Build history of the part. All positions in model axes, mm. A direction names the side the tool comes from. Coordinates: 2 decimals unless noted, no trailing zeros. Write each loop counter-clockwise with the first axis right and the second up, starting at its lowest first coordinate (ties: lowest second). Pieces come first, ordered by that corner, then holes. Notation, with made-up numbers: (-31.75, 19) -> (0.25, 19) arc R20 ccw to (0.25, 39) -> close; hole circle Ø7 at (-36, -9). An arc over 180 degrees is marked (long way). Write each question's results on one line, items separated by ' | '. Start each with the question number.
Q1. Saw through at B-B on z = 31. Give the cut face in (x, y), and give its area (3 significant figures).
Q2. Drop a flat-ended pin along its axis: pin 1 Ø8 at (x, z) = (22, -3) entering from -Y. Give the stop position or say it passes through.
Q3. Two-plate mould, pull along Z, no slides. Class faces 1 (the face through (-18.07, 1.48, -27.26)), 2 (the face through (-43, 26, -43)), 3 (the face through (-41, 29, 41)): released by +Z, released by -Z, zero draft, split by the parting line, or undercut.
Q4. Tool access for faces 4 (the face through (39.3, 27.5, -40.8)), 5 (the face through (-18.583, 1.479, 27.776)), 6 (the face through (-27.776, 1.479, -18.583)): list every direction of +Z, -Z, +X, -X, +Y, -Y with a clear straight run to the whole face (end or side of a thin tool).
Q5. Saw through at C-C on x = 41.25. Give the cut face in (y, z), and give its area (3 significant figures).
Q6. Drill centre lines: line 1 (Z direction, x = -41, y = 3.75); line 2 (Y direction, x = -14, z = 5); line 3 (X direction, y = 19.75, z = -40.5). Where is each one in solid material? Low to high.
Q7. Saw through at A-A on x = 26. Give the cut face in (y, z).
Q8. Saw through at D-D on z = -41.25. Give the cut face in (x, y), and give its area (3 significant figures).
Autodesk Inventor part; units mm, degrees
ref_plane "YZ Plane" through (0, 0, 0) normal (1, 0, 0) x (0, 1, 0)
ref_plane "XZ Plane" through (0, 0, 0) normal (0, 1, 0) x (-1, 0, 0)
ref_plane "XY Plane" through (0, 0, 0) normal (0, 0, 1) x (1, 0, 0)
sketch "Sketch1" plane through (0, 0, 0) normal (0, 1, 0) x (-1, 0, 0)
  line L0 (41.25, -41.25) -> (-41.25, -41.25) construction
  line L1 (-41.25, -41.25) -> (-41.25, 41.25) construction
  line L2 (-41.25, 41.25) -> (41.25, 41.25) construction
  line L3 (41.25, 41.25) -> (41.25, -41.25) construction
  circle A0 centre (41.25, -41.25) radius 3.5
  circle A1 centre (41.25, -41.25) radius 2
  circle A2 centre (41.25, -41.25) radius 6.5
  line L4 (45.8462, -36.6538) -> (4.5962, 4.5962)
  line L5 (4.5962, 4.5962) -> (-4.5962, -4.5962)
  line L6 (-4.5962, -4.5962) -> (36.6538, -45.8462)
  point P0 (0, 0)
  point P1 (0, -41.25)
  point P2 (-41.25, 0)
  point P3 (0, 0)
  dimension "d0" = 82.5
  dimension "d1" = 4
  dimension "d2" = 7
  dimension "d3" = 3
extrude "Extrusion1" add sketch "Sketch1" along normal blind 3 contours A2 L6 L5 L4
extrude "Extrusion2" add sketch "Sketch1" along normal blind 29 contours A1
extrude "Extrusion3" add sketch "Sketch1" along normal blind 26 contours A0
extrude "Extrusion4" add sketch "Sketch1" along normal blind 3 contours A2
pattern_circular "Circular Pattern1" count 4 over 360 about axis through (0, -10, 0) along (0, 1, 0) of "Extrusion1", "Extrusion2", "Extrusion3", "Extrusion4"
properties part number "ConformalCoatingJig_3DPrint"
Returned:
1) outline: (-40.19, 0) -> (-21.81, 0) -> (-21.81, 3) -> (-40.19, 3) -> close; (21.81, 0) -> (40.19, 0) -> (40.19, 3) -> (21.81, 3) -> close | area: 110 mm2
2) pin 1: passes through
3) face 1: released by -Z | face 2: undercut | face 3: zero draft
4) face 4: +Y | face 5: +Z, +Y, -Y | face 6: -X, +Y, -Y
5) outline: (0, -47.75) -> (3, -47.75) -> (3, -44.75) -> (26, -44.75) -> (26, -43.25) -> (29, -43.25) -> (29, -39.25) -> (26, -39.25) -> (26, -37.75) -> (3, -37.75) -> (3, -32.06) -> (0, -32.06) -> close; (0, 32.06) -> (3, 32.06) -> (3, 37.75) -> (26, 37.75) -> (26, 39.25) -> (29, 39.25) -> (29, 43.25) -> (26, 43.25) -> (26, 44.75) -> (3, 44.75) -> (3, 47.75) -> (0, 47.75) -> close | area: 440 mm2
6) line 1: z = -44.74 to -37.76, 37.76 to 44.74 | line 2: y = 0 to 3 | line 3: x = -44.67 to -37.83, 37.83 to 44.67
7) outline: (0, -35.19) -> (3, -35.19) -> (3, -16.81) -> (0, -16.81) -> close; (0, 16.81) -> (3, 16.81) -> (3, 35.19) -> (0, 35.19) -> close
8) outline: (-47.75, 0) -> (-32.06, 0) -> (-32.06, 3) -> (-37.75, 3) -> (-37.75, 26) -> (-39.25, 26) -> (-39.25, 29) -> (-43.25, 29) -> (-43.25, 26) -> (-44.75, 26) -> (-44.75, 3) -> (-47.75, 3) -> close; (32.06, 0) -> (47.75, 0) -> (47.75, 3) -> (44.75, 3) -> (44.75, 26) -> (43.25, 26) -> (43.25, 29) -> (39.25, 29) -> (39.25, 26) -> (37.75, 26) -> (37.75, 3) -> (32.06, 3) -> close | area: 440 mm2
